Read the model definition and answer for the solid it produces. Units are mm, in the model's axes. Face numbers are marked on the shaded views. A direction names the side the tool comes from. Coordinates: 2 decimals unless noted, no trailing zeros. Write each loop counter-clockwise with the first axis right and the second up, starting at its lowest first coordinate (ties: lowest second). Pieces come first, ordered by that corner, then holes. Notation, with made-up numbers: (74, -3.5) -> (81, -3.5) arc R15 cw to (81, 20.5) -> close; hole circle Ø6 at (4.5, 49). An arc over 180 degrees is marked (long way). Return JSON: item names as keys, results as strings.
from build123d import *

# Parameters (mm, degrees)
SKETCH1_W           = 139.7
SKETCH1_H           = 76.2
BOSS_EXTRUDE1_DEPTH = 6.35
SKETCH2_W           = 139.7
SKETCH2_H           = 12.7
BOSS_EXTRUDE2_DEPTH = 19.05
SKETCH3_R           = 2.032
CUT_EXTRUDE1_DEPTH  = 82.814026915
CUT_EXTRUDE2_DEPTH  = 3.048
SKETCH5_R           = 3.175
BOSS_EXTRUDE3_DEPTH = 6.35


with BuildPart() as part:
    # Sketch1 → Boss-Extrude1 (new body)
    with BuildSketch(Plane(origin=(0, 0, 0), x_dir=(1, 0, 0), z_dir=(0, 1, 0))):
        Rectangle(SKETCH1_W, SKETCH1_H)
    extrude(amount=BOSS_EXTRUDE1_DEPTH)

    # Sketch2 → Boss-Extrude2 (add)
    with BuildSketch(Plane(origin=(0, 6.35, 0), x_dir=(1, 0, 0), z_dir=(0, 1, 0))):
        with Locations((0, -31.75)):
            Rectangle(SKETCH2_W, SKETCH2_H)
    extrude(amount=BOSS_EXTRUDE2_DEPTH)

    # Sketch3 → Cut-Extrude1 (cut, through all)
    with BuildSketch(Plane(origin=(0, 6.35, 0), x_dir=(1, 0, 0), z_dir=(0, 1, 0))):
        with Locations(Location((-53.34, -21.59, 0), (0, 0, 270))):
            Circle(SKETCH3_R)
    extrude(amount=-CUT_EXTRUDE1_DEPTH, mode=Mode.SUBTRACT)

    # Sketch4 → Cut-Extrude2 (cut)
    with BuildSketch(Plane.XZ):
        Polygon((-50.927, 25.769438599), (-55.753, 25.769438599), (-58.166, 21.59), (-55.753, 17.410561401), (-50.927, 17.410561401), (-48.514, 21.59), align=None)
    extrude(amount=-CUT_EXTRUDE2_DEPTH, mode=Mode.SUBTRACT)

    # Sketch5 → Boss-Extrude3 (add)
    with BuildSketch(Plane(origin=(0, 25.4, 0), x_dir=(1, 0, 0), z_dir=(0, 1, 0))):
        with Locations(Location((-57.15, -31.75, 0), (0, 0, 270))):
            Circle(SKETCH5_R)
        with Locations(Location((0, -31.75, 0), (0, 0, 270))):
            Circle(SKETCH5_R)
        with Locations(Location((57.15, -31.75, 0), (0, 0, 270))):
            Circle(SKETCH5_R)
    extrude(amount=BOSS_EXTRUDE3_DEPTH)


solid = part.part
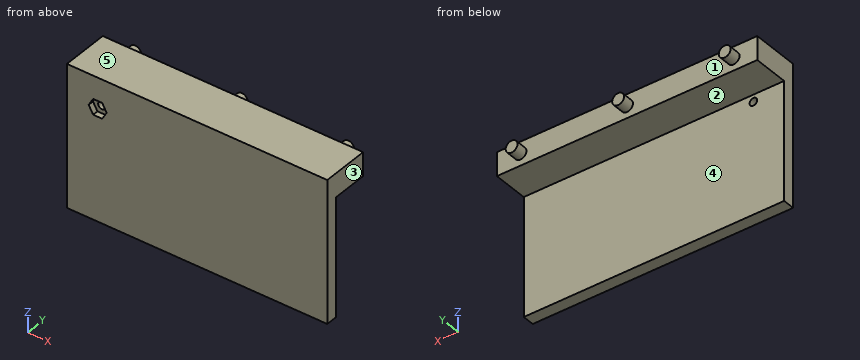
1. The part is cut by section B-B (x = 57.15). Determine the outline of the cut face in (y, z) (3 decimals), then the cut area to 3 significant figures.
Taken from the geometry:
{"outline": "(0, -38.1) -> (6.35, -38.1) -> (6.35, 25.4) -> (25.4, 25.4) -> (25.4, 28.575) -> (31.75, 28.575) -> (31.75, 34.925) -> (25.4, 34.925) -> (25.4, 38.1) -> (0, 38.1) -> close", "area": "766 mm2"}
2. The part is cut by section A-A (z = 31.75). Determine the outline of the cut face in (x, y) (3 decimals), then the cut area to 3 significant figures.
Taken from the geometry:
{"outline": "(-69.85, 0) -> (69.85, 0) -> (69.85, 25.4) -> (60.325, 25.4) -> (60.325, 31.75) -> (53.975, 31.75) -> (53.975, 25.4) -> (3.175, 25.4) -> (3.175, 31.75) -> (-3.175, 31.75) -> (-3.175, 25.4) -> (-53.975, 25.4) -> (-53.975, 31.75) -> (-60.325, 31.75) -> (-60.325, 25.4) -> (-69.85, 25.4) -> close", "area": "3,670 mm2"}
3. For a pull along X with two mould halves and no side action, classify the marked faces 1, 2 and 3 as +X half, -X half, draft (parallel to the pull), parting line (faces both ways), or undercut.
Taken from the geometry:
{"face 1": "undercut", "face 2": "draft", "face 3": "+X half"}
4. Consider L1, parallel to Z at x = -53, y = 5; L2, parallel to X at y = 4.9, z = 21.59; L3, parallel to Z at x = 33.5, y = 19. Determine where each line is inside the solid, lowest interval first.
Taken from the geometry:
{"L1": "z = -38.1 to 19.59, 23.59 to 38.1", "L2": "x = -69.85 to -55.37, -51.31 to 69.85", "L3": "z = 25.4 to 38.1"}
5. The part is cut by section C-C (y = 28). Determine the outline of the cut face in (x, z) (3 decimals).
Taken from the geometry:
{"outline": "circle Ø6.35 at (-57.15, 31.75); circle Ø6.35 at (0, 31.75); circle Ø6.35 at (57.15, 31.75)"}
6. Flat-ended cylindrical pins translate along their axes: pin 1 Ø5 at (x, z) = (53, 25.5) entering from +Y; pin 2 Ø8 at (x, z) = (-32.5, -13.5) entering from +Y; pin 3 Ø9 at (x, z) = (-52.5, 23) entering from -Y; pin 4 Ø5.5 at (x, y) = (10, 15) entering from -Z. Find the tip coordinate at first contact, or state that the pin passes through.
Taken from the geometry:
{"pin 1": "stops at y = 25.4", "pin 2": "stops at y = 6.35", "pin 3": "stops at y = 0", "pin 4": "stops at z = 25.4"}
7. The part is cut by section D-D (x = -17.5). Determine the outline of the cut face in (y, z), then the cut area to 3 significant figures.
Taken from the geometry:
{"outline": "(0, -38.1) -> (6.35, -38.1) -> (6.35, 25.4) -> (25.4, 25.4) -> (25.4, 38.1) -> (0, 38.1) -> close", "area": "726 mm2"}
8. A tool of negligible diameter and unlimited length cuts with its end or side. For the marked faces 4 and 5, from which of +Z, -Z, +X, -X, +Y, -Y can it reach the whole face along a straight path? Write none if from no direction.
Taken from the geometry:
{"face 4": "-Z, +X, -X, +Y", "face 5": "+Z, +X, -X, +Y, -Y"}
